CAD build for the part. Positions are in the model's coordinates, mm. A direction names the side the tool comes from. Round coordinates to 2 decimals unless told otherwise and drop trailing zeros. Write each loop counter-clockwise with the first axis right and the second up, starting at its lowest first coordinate (ties: lowest second). Pieces come first, ordered by that corner, then holes. Notation, with made-up numbers: (59, 89.25) -> (65, 89.25) arc R11 cw to (65, 110.25) -> close; hole circle Ø6 at (12, 12.25). An arc over 180 degrees is marked (long way). Put each result on its own line as item: value. Start each with the question number.
1. Saw through at B-B on x = 1. List the corners of the cut face in (y, z).
2. 3-axis set-ups, long thin cutter, end or side, ignore diameter. For faces 4 (the flat face through (-15, 2, -5.169)), 5 (the flat face through (28, 2, -5.169)), 6 (the flat face through (28, 2, 1.031)), 7 (the flat face through (28, 3.7, -2)), 8 (the flat face through (29.301, 2, -2)): which of +Z, -Z, +X, -X, +Y, -Y reach the whole face in a straight line?
3. Saw through at A-A on z = -6. List the corners of the cut face in (x, y), and give its area (3 significant figures).
4. Saw through at C-C on z = 4.5. List the corners of the cut face in (x, y), and give its area (3 significant figures).
5. Flat gauge pins, fed straight in: P1, Ø6, axis at x = 21.5, z = -1, coming from the -Y side; P2, Ø6, axis at y = 10, z = -3, coming from the -X side; P3, Ø0.8, axis at x = 27.5, z = -1.5, coming from the +Y side; P4, Ø1.2, axis at x = -15, y = 1, coming from the -Z side. Where does each tip first touch, or does it go through?
6. Pull direction Y, two halves, no side cores. Call faces 1 (the cylindrical face through (-1.53, 42.17, -3.22)), 2 (the flat face through (30, 31.9, -2)), 3 (the flat face through (26.801, 15, -2)): pulls with the +Y half, pulls with the -Y half, needs draft (parallel to the pull), parting line crosses it, or undercut.
7. Saw through at D-D on y = 28. List the corners of the cut face in (x, z), and give its area (3 significant figures).
8. Drill centre lines: line 1 (Y direction, x = 27.5, z = -0.75); line 2 (X direction, y = 32.5, z = 6.25); line 3 (X direction, y = 3, z = 0). Where is each one in solid material? Low to high. Write a range as from..to.
Autodesk Inventor part; units mm, degrees
ref_plane "YZ Plane" through (0, 0, 0) normal (1, 0, 0) x (0, 1, 0)
ref_plane "XZ Plane" through (0, 0, 0) normal (0, 1, 0) x (-1, 0, 0)
ref_plane "XY Plane" through (0, 0, 0) normal (0, 0, 1) x (1, 0, 0)
sketch "Sketch1" plane through (0, 0, 0) normal (0, 1, 0) x (-1, 0, 0)
  line L0 (13.3986, -11.7687) -> (-26.8014, -11.7687)
  line L1 (-26.8014, -11.7687) -> (-26.8014, 7.6313)
  line L2 (-26.8014, 7.6313) -> (13.3986, 7.6313)
  line L3 (13.3986, 7.6313) -> (13.3986, -11.7687)
  point P0 (0, 0)
  dimension "d0" = 19.4
  dimension "d1" = 40.2
extrude "Extrusion1" add sketch "Sketch1" along normal blind 39.7
sketch "Sketch2" plane through (26.8014, 0, 7.6313) normal (1, 0, 0) x (0, 0, -1)
  line L0 (6.6, 3.7) -> (12.8, 3.7)
  line L1 (12.8, 3.7) -> (12.8, 0)
  line L2 (12.8, 0) -> (6.6, 0)
  line L3 (6.6, 0) -> (6.6, 3.7)
  line L4 (19.4, 0) -> (19.4, 39.7)
  line L5 (0, 0) -> (0, 39.7)
  line L6 (0, 0) -> (19.4, 0)
  point P0 (7.6313, 0)
  point P1 (12.8, 1.85)
  point P2 (6.6, 1.85)
  dimension "d4" = 6.2
  dimension "d5" = 3.7
  dimension "d6" = 6.6
  dimension "d7" = 6.6
  dimension "d8" = 0
extrude "Extrusion2" add sketch "Sketch2" along normal blind 2.5
sketch "Sketch5" plane through (-13.3986, 0, -11.7687) normal (-1, 0, 0) x (0, 0, 1)
  line L0 (6.6, 3.7) -> (12.8, 3.7)
  line L1 (6.6, 3.7) -> (12.8, 3.7)
  line L2 (12.8, 3.7) -> (12.8, 0)
  line L3 (12.8, 0) -> (6.6, 0)
  line L4 (6.6, 0) -> (6.6, 3.7)
  point P0 (11.7687, 0)
extrude "Extrusion3" add sketch "Sketch5" along normal blind 2.5
sketch "Sketch6" plane through (26.8014, 0, -11.7687) normal (1, 0, 0) x (0, 0, -1)
  line L0 (-19.4, 0) -> (-19.4, 39.7)
  line L1 (0, 0) -> (0, 39.7)
  line L2 (-19.4, 31.9) -> (0, 31.9)
  line L3 (0, 31.9) -> (0, 29.8)
  line L4 (0, 29.8) -> (-19.4, 29.8)
  line L5 (-19.4, 29.8) -> (-19.4, 31.9)
  line L6 (-19.4, 39.7) -> (0, 39.7)
  point P0 (-11.7687, 0)
  point P1 (0, 31.9)
  dimension "d13" = 2.1
  dimension "d14" = 7.8
extrude "Extrusion4" add sketch "Sketch6" along normal blind 7 contours L0 L2 L1 L4
sketch "Sketch7" plane through (-13.3986, 0, 7.6313) normal (-1, 0, 0) x (0, 0, 1)
  line L0 (-19.4, 29.8) -> (-19.4, 31.9)
  line L1 (-19.4, 29.8) -> (-19.4, 31.9)
  line L2 (0, 31.9) -> (0, 29.8)
  line L3 (-19.4, 31.9) -> (0, 31.9)
  line L4 (0, 31.9) -> (0, 29.8)
  line L5 (0, 29.8) -> (-19.4, 29.8)
  point P0 (-7.6313, 0)
extrude "Extrusion5" add sketch "Sketch7" along normal blind 7
sketch "Sketch8" plane through (0, 39.7, 0) normal (0, 1, 0) x (1, 0, 0)
  circle A0 centre (8.4014, 2.0687) radius 5.5
  line L0 (26.8014, -7.6313) -> (26.8014, 11.7687)
  line L1 (26.8014, 11.7687) -> (-13.3986, 11.7687)
  point P0 (0, 0)
  dimension "d19" = 11
  dimension "d20" = 18.4
  dimension "d23" = 9.7
extrude "Extrusion6" add sketch "Sketch8" along normal blind 2
sketch "Sketch10" plane through (0, 39.7, 0) normal (0, 1, 0) x (1, 0, 0)
  circle A0 centre (-4.2986, 2.0687) radius 3
  line L0 (-13.3986, 11.7687) -> (-13.3986, -7.6313)
  point P0 (0, 0)
  dimension "d26" = 6
  dimension "d27" = 9.1
extrude "Extrusion7" add sketch "Sketch10" along normal blind 5
sketch "Sketch11" plane through (26.8014, 31.9, 7.6313) normal (0, 1, 0) x (1, 0, 0)
  circle A0 centre (3.2, 5) radius 2.7
  line L0 (0, 0) -> (7, 0)
  circle A1 centre (3.2, 14.4) radius 2.7
  line L1 (0, 19.4) -> (7, 19.4)
  line L2 (0, 0) -> (0, 19.4)
  line L3 (7, 19.4) -> (7, 0)
  point P0 (-26.8014, 7.6313)
  dimension "d30" = 5.4
  dimension "d31" = 5
  dimension "d32" = 5
  dimension "d33" = 5.4
  dimension "d38" = 3.8
  dimension "d39" = 3.8
extrude "Extrusion8" cut sketch "Sketch11" against normal blind 5 contours A0 | A1
sketch "Sketch12" plane through (-13.3986, 31.9, 7.6313) normal (0, 1, 0) x (1, 0, 0)
  circle A0 centre (-3.2, 14.4) radius 2.7
  circle A1 centre (-3.2, 5) radius 2.7
  line L0 (0, 0) -> (-7, 0)
  line L1 (0, 19.4) -> (-7, 19.4)
  line L2 (-7, 0) -> (-7, 19.4)
  point P0 (13.3986, 7.6313)
  dimension "d42" = 5.4
  dimension "d43" = 5.4
  dimension "d44" = 5
  dimension "d45" = 5
  dimension "d46" = 3.8
  dimension "d47" = 3.8
extrude "Extrusion9" cut sketch "Sketch12" against normal blind 7
equation "\"d31\" = d32"
equation "\"d33\" = d30"
equation "\"d39\" = d38"
equation "\"d43\" = d42"
equation "\"d45\" = d44"
equation "\"d47\" = d46"
properties part number "Servo"
Return value:
1. outline: (0, -11.77) -> (39.7, -11.77) -> (39.7, 7.63) -> (0, 7.63) -> close
2. face 4: -Z, -X, -Y
2. face 5: -Z, +X, -Y
2. face 6: +Z, +X, -Y
2. face 7: +Z, -Z, +X
2. face 8: +Z, -Z, +X, -Y
3. outline: (-20.4, 29.8) -> (-19.19, 29.8) -> (-19.19, 31.9) -> (-20.4, 31.9) -> close; (-14.01, 29.8) -> (-13.4, 29.8) -> (-13.4, 0) -> (26.8, 0) -> (26.8, 29.8) -> (27.41, 29.8) -> (27.41, 31.9) -> (26.8, 31.9) -> (26.8, 39.7) -> (12.25, 39.7) -> (12.25, 41.7) -> (4.55, 41.7) -> (4.55, 39.7) -> (-13.4, 39.7) -> (-13.4, 31.9) -> (-14.01, 31.9) -> close; (32.59, 29.8) -> (33.8, 29.8) -> (33.8, 31.9) -> (32.59, 31.9) -> close
3. area: 1,620 mm^2
4. outline: (-20.4, 29.8) -> (-18.55, 29.8) -> (-18.55, 31.9) -> (-20.4, 31.9) -> close; (-14.65, 29.8) -> (-13.4, 29.8) -> (-13.4, 0) -> (26.8, 0) -> (26.8, 29.8) -> (28.05, 29.8) -> (28.05, 31.9) -> (26.8, 31.9) -> (26.8, 39.7) -> (-13.4, 39.7) -> (-13.4, 31.9) -> (-14.65, 31.9) -> close; (31.95, 29.8) -> (33.8, 29.8) -> (33.8, 31.9) -> (31.95, 31.9) -> close
4. area: 1,610 mm^2
5. P1: stops at y = 0
5. P2: stops at x = -13.4
5. P3: stops at y = 31.9
5. P4: stops at z = -5.17
6. face 1: needs draft
6. face 2: pulls with the +Y half
6. face 3: undercut
7. outline: (-13.4, -11.77) -> (26.8, -11.77) -> (26.8, 7.63) -> (-13.4, 7.63) -> close
7. area: 780 mm^2
8. line 1: y = 0..3.7, 29.8..31.9
8. line 2: x = -13.4..26.8
8. line 3: x = -15.9..29.3
